Here's how the part is built. I have some questions about the finished solid (model axes, mm). A direction names the side the tool comes from. Round coordinates to 2 decimals unless told otherwise and drop trailing zeros. Order: outer loops, then holes, each group sorted by start corner. A loop starts at its lowest first (then second) coordinate and runs counter-clockwise, first axis right, second up.
```python
from build123d import *

# Parameters (mm, degrees)
SKETCH_1_W          = 350
SKETCH_1_H          = 50
SKETCH_1_R          = 2.75
EXTRUDE_1_DEPTH     = 5
SKETCH_2_W          = 350
SKETCH_2_H          = 6
EXTRUDE_2_DEPTH     = 364
SKETCH_3_R          = 2.75
CUT_EXTRUDE_1_DEPTH = 500
SKETCH_4_R          = 1.75
CUT_EXTRUDE_2_DEPTH = 10
FILLET_1_R          = 20
SKETCH_5_R          = 1.75
CUT_EXTRUDE_3_DEPTH = 10


with BuildPart() as part:
    # 草图1 → 凸台-拉伸1 (new body)
    with BuildSketch(Plane(origin=(0, 0, 0), x_dir=(1, 0, 0), z_dir=(0, 1, 0))):
        with Locations((0, 25)):
            Rectangle(SKETCH_1_W, SKETCH_1_H)
        with Locations(Location((130, 25, 0), (0, 0, 270))):
            Circle(SKETCH_1_R, mode=Mode.SUBTRACT)
        with Locations(Location((50, 25, 0), (0, 0, 270))):
            Circle(SKETCH_1_R, mode=Mode.SUBTRACT)
        with Locations(Location((-130, 25, 0), (0, 0, 90))):
            Circle(SKETCH_1_R, mode=Mode.SUBTRACT)
        with Locations(Location((-50, 25, 0), (0, 0, 90))):
            Circle(SKETCH_1_R, mode=Mode.SUBTRACT)
    extrude(amount=EXTRUDE_1_DEPTH)

    # 草图2 → 凸台-拉伸2 (add)
    with BuildSketch(Plane(origin=(0, 5, 0), x_dir=(1, 0, 0), z_dir=(0, 1, 0))):
        with Locations((0, 3)):
            Rectangle(SKETCH_2_W, SKETCH_2_H)
    extrude(amount=EXTRUDE_2_DEPTH)

    # 草图3 → 切除-拉伸1 (cut)
    with BuildSketch(Plane(origin=(0, 0, -6), x_dir=(-1, 0, 0), z_dir=(0, 0, -1))):
        with Locations((87.5, 274)):
            Circle(SKETCH_3_R)
        with Locations((87.5, 124)):
            Circle(SKETCH_3_R)
        with Locations((-87.5, 124)):
            Circle(SKETCH_3_R)
        with Locations((-87.5, 274)):
            Circle(SKETCH_3_R)
        with Locations((152.5, 339)):
            Circle(SKETCH_3_R)
        with Locations((152.5, 189)):
            Circle(SKETCH_3_R)
        with Locations((152.5, 39)):
            Circle(SKETCH_3_R)
        with Locations((-152.5, 39)):
            Circle(SKETCH_3_R)
        with Locations((-152.5, 189)):
            Circle(SKETCH_3_R)
        with Locations((-152.5, 339)):
            Circle(SKETCH_3_R)
        with Locations((0, 339)):
            Circle(SKETCH_3_R)
        with Locations((0, 189)):
            Circle(SKETCH_3_R)
        with Locations((0, 39)):
            Circle(SKETCH_3_R)
        with BuildLine():
            Line((83.964466094, 137.535533906), (41.035533906, 180.464466094))
            ThreePointArc((41.035533906, 180.464466094), (39.951670149, 185.913417162), (44.571067812, 189))
            Line((44.571067812, 189), (130.428932188, 189))
            ThreePointArc((130.428932188, 189), (135.048329851, 185.913417162), (133.964466094, 180.464466094))
            Line((133.964466094, 180.464466094), (91.035533906, 137.535533906))
            ThreePointArc((91.035533906, 137.535533906), (87.5, 136.071067812), (83.964466094, 137.535533906))
        make_face()
        with BuildLine():
            Line((44.571067812, 339), (130.428932188, 339))
            ThreePointArc((130.428932188, 339), (135.048329851, 335.913417162), (133.964466094, 330.464466094))
            Line((133.964466094, 330.464466094), (91.035533906, 287.535533906))
            ThreePointArc((91.035533906, 287.535533906), (87.5, 286.071067812), (83.964466094, 287.535533906))
            Line((83.964466094, 287.535533906), (41.035533906, 330.464466094))
            ThreePointArc((41.035533906, 330.464466094), (39.951670149, 335.913417162), (44.571067812, 339))
        make_face()
        with BuildLine():
            Line((73.964466094, 120.464466094), (31.035533906, 77.535533906))
            ThreePointArc((31.035533906, 77.535533906), (25.586582838, 76.451670149), (22.5, 81.071067812))
            Line((22.5, 81.071067812), (22.5, 166.928932188))
            ThreePointArc((22.5, 166.928932188), (25.586582838, 171.548329851), (31.035533906, 170.464466094))
            Line((31.035533906, 170.464466094), (73.964466094, 127.535533906))
            ThreePointArc((73.964466094, 127.535533906), (75.428932188, 124), (73.964466094, 120.464466094))
        make_face()
        with BuildLine():
            Line((101.035533906, 277.535533906), (143.964466094, 320.464466094))
            ThreePointArc((143.964466094, 320.464466094), (149.413417162, 321.548329851), (152.5, 316.928932188))
            Line((152.5, 316.928932188), (152.5, 231.071067812))
            ThreePointArc((152.5, 231.071067812), (149.413417162, 226.451670149), (143.964466094, 227.535533906))
            Line((143.964466094, 227.535533906), (101.035533906, 270.464466094))
            ThreePointArc((101.035533906, 270.464466094), (99.571067812, 274), (101.035533906, 277.535533906))
        make_face()
        with BuildLine():
            Line((91.035533906, 260.464466094), (133.964466094, 217.535533906))
            ThreePointArc((133.964466094, 217.535533906), (135.048329851, 212.086582838), (130.428932188, 209))
            Line((130.428932188, 209), (44.571067812, 209))
            ThreePointArc((44.571067812, 209), (39.951670149, 212.086582838), (41.035533906, 217.535533906))
            Line((41.035533906, 217.535533906), (83.964466094, 260.464466094))
            ThreePointArc((83.964466094, 260.464466094), (87.5, 261.928932188), (91.035533906, 260.464466094))
        make_face()
        with BuildLine():
            Line((73.964466094, 270.464466094), (31.035533906, 227.535533906))
            ThreePointArc((31.035533906, 227.535533906), (25.586582838, 226.451670149), (22.5, 231.071067812))
            Line((22.5, 231.071067812), (22.5, 316.928932188))
            ThreePointArc((22.5, 316.928932188), (25.586582838, 321.548329851), (31.035533906, 320.464466094))
            Line((31.035533906, 320.464466094), (73.964466094, 277.535533906))
            ThreePointArc((73.964466094, 277.535533906), (75.428932188, 274), (73.964466094, 270.464466094))
        make_face()
        with BuildLine():
            Line((101.035533906, 127.535533906), (143.964466094, 170.464466094))
            ThreePointArc((143.964466094, 170.464466094), (149.413417162, 171.548329851), (152.5, 166.928932188))
            Line((152.5, 166.928932188), (152.5, 81.071067812))
            ThreePointArc((152.5, 81.071067812), (149.413417162, 76.451670149), (143.964466094, 77.535533906))
            Line((143.964466094, 77.535533906), (101.035533906, 120.464466094))
            ThreePointArc((101.035533906, 120.464466094), (99.571067812, 124), (101.035533906, 127.535533906))
        make_face()
        with BuildLine():
            Line((91.035533906, 110.464466094), (133.964466094, 67.535533906))
            ThreePointArc((133.964466094, 67.535533906), (135.048329851, 62.086582838), (130.428932188, 59))
            Line((130.428932188, 59), (44.571067812, 59))
            ThreePointArc((44.571067812, 59), (39.951670149, 62.086582838), (41.035533906, 67.535533906))
            Line((41.035533906, 67.535533906), (83.964466094, 110.464466094))
            ThreePointArc((83.964466094, 110.464466094), (87.5, 111.928932188), (91.035533906, 110.464466094))
        make_face()
        with BuildLine():
            Line((-91.035533906, 137.535533906), (-133.964466094, 180.464466094))
            ThreePointArc((-133.964466094, 180.464466094), (-135.048329851, 185.913417162), (-130.428932188, 189))
            Line((-130.428932188, 189), (-44.571067812, 189))
            ThreePointArc((-44.571067812, 189), (-39.951670149, 185.913417162), (-41.035533906, 180.464466094))
            Line((-41.035533906, 180.464466094), (-83.964466094, 137.535533906))
            ThreePointArc((-83.964466094, 137.535533906), (-87.5, 136.071067812), (-91.035533906, 137.535533906))
        make_face()
        with BuildLine():
            Line((-101.035533906, 120.464466094), (-143.964466094, 77.535533906))
            ThreePointArc((-143.964466094, 77.535533906), (-149.413417162, 76.451670149), (-152.5, 81.071067812))
            Line((-152.5, 81.071067812), (-152.5, 166.928932188))
            ThreePointArc((-152.5, 166.928932188), (-149.413417162, 171.548329851), (-143.964466094, 170.464466094))
            Line((-143.964466094, 170.464466094), (-101.035533906, 127.535533906))
            ThreePointArc((-101.035533906, 127.535533906), (-99.571067812, 124), (-101.035533906, 120.464466094))
        make_face()
        with BuildLine():
            Line((-73.964466094, 127.535533906), (-31.035533906, 170.464466094))
            ThreePointArc((-31.035533906, 170.464466094), (-25.586582838, 171.548329851), (-22.5, 166.928932188))
            Line((-22.5, 166.928932188), (-22.5, 81.071067812))
            ThreePointArc((-22.5, 81.071067812), (-25.586582838, 76.451670149), (-31.035533906, 77.535533906))
            Line((-31.035533906, 77.535533906), (-73.964466094, 120.464466094))
            ThreePointArc((-73.964466094, 120.464466094), (-75.428932188, 124), (-73.964466094, 127.535533906))
        make_face()
        with BuildLine():
            Line((-83.964466094, 110.464466094), (-41.035533906, 67.535533906))
            ThreePointArc((-41.035533906, 67.535533906), (-39.951670149, 62.086582838), (-44.571067812, 59))
            Line((-44.571067812, 59), (-130.428932188, 59))
            ThreePointArc((-130.428932188, 59), (-135.048329851, 62.086582838), (-133.964466094, 67.535533906))
            Line((-133.964466094, 67.535533906), (-91.035533906, 110.464466094))
            ThreePointArc((-91.035533906, 110.464466094), (-87.5, 111.928932188), (-83.964466094, 110.464466094))
        make_face()
        with BuildLine():
            Line((-91.035533906, 287.535533906), (-133.964466094, 330.464466094))
            ThreePointArc((-133.964466094, 330.464466094), (-135.048329851, 335.913417162), (-130.428932188, 339))
            Line((-130.428932188, 339), (-44.571067812, 339))
            ThreePointArc((-44.571067812, 339), (-39.951670149, 335.913417162), (-41.035533906, 330.464466094))
            Line((-41.035533906, 330.464466094), (-83.964466094, 287.535533906))
            ThreePointArc((-83.964466094, 287.535533906), (-87.5, 286.071067812), (-91.035533906, 287.535533906))
        make_face()
        with BuildLine():
            Line((-101.035533906, 270.464466094), (-143.964466094, 227.535533906))
            ThreePointArc((-143.964466094, 227.535533906), (-149.413417162, 226.451670149), (-152.5, 231.071067812))
            Line((-152.5, 231.071067812), (-152.5, 316.928932188))
            ThreePointArc((-152.5, 316.928932188), (-149.413417162, 321.548329851), (-143.964466094, 320.464466094))
            Line((-143.964466094, 320.464466094), (-101.035533906, 277.535533906))
            ThreePointArc((-101.035533906, 277.535533906), (-99.571067812, 274), (-101.035533906, 270.464466094))
        make_face()
        with BuildLine():
            Line((-73.964466094, 277.535533906), (-31.035533906, 320.464466094))
            ThreePointArc((-31.035533906, 320.464466094), (-25.586582838, 321.548329851), (-22.5, 316.928932188))
            Line((-22.5, 316.928932188), (-22.5, 231.071067812))
            ThreePointArc((-22.5, 231.071067812), (-25.586582838, 226.451670149), (-31.035533906, 227.535533906))
            Line((-31.035533906, 227.535533906), (-73.964466094, 270.464466094))
            ThreePointArc((-73.964466094, 270.464466094), (-75.428932188, 274), (-73.964466094, 277.535533906))
        make_face()
        with BuildLine():
            Line((-83.964466094, 260.464466094), (-41.035533906, 217.535533906))
            ThreePointArc((-41.035533906, 217.535533906), (-39.951670149, 212.086582838), (-44.571067812, 209))
            Line((-44.571067812, 209), (-130.428932188, 209))
            ThreePointArc((-130.428932188, 209), (-135.048329851, 212.086582838), (-133.964466094, 217.535533906))
            Line((-133.964466094, 217.535533906), (-91.035533906, 260.464466094))
            ThreePointArc((-91.035533906, 260.464466094), (-87.5, 261.928932188), (-83.964466094, 260.464466094))
        make_face()
    extrude(amount=-CUT_EXTRUDE_1_DEPTH, mode=Mode.SUBTRACT)

    # 草图4 → 切除-拉伸2 (cut)
    with BuildSketch(Plane.XY):
        with Locations((60, 366)):
            Circle(SKETCH_4_R)
        with Locations((85, 366)):
            Circle(SKETCH_4_R)
        with Locations((12.5, 366)):
            Circle(SKETCH_4_R)
        with Locations((-12.5, 366)):
            Circle(SKETCH_4_R)
        with Locations((-85, 366)):
            Circle(SKETCH_4_R)
        with Locations((-60, 366)):
            Circle(SKETCH_4_R)
    extrude(amount=-CUT_EXTRUDE_2_DEPTH, mode=Mode.SUBTRACT)

    # 圆角1
    fillet_1_edges = [part.edges().sort_by_distance(p)[0] for p in [
        (-175, 369, -3),
        (175, 369, -3),
    ]]
    fillet(fillet_1_edges, radius=FILLET_1_R)

    # 草图5 → 切除-拉伸3 (cut)
    with BuildSketch(Plane(origin=(0, 0, -6), x_dir=(-1, 0, 0), z_dir=(0, 0, -1))):
        with Locations((172, 330)):
            Circle(SKETCH_5_R)
        with Locations((172, 230)):
            Circle(SKETCH_5_R)
        with Locations((-172, 230)):
            Circle(SKETCH_5_R)
        with Locations((-172, 330)):
            Circle(SKETCH_5_R)
    extrude(amount=-CUT_EXTRUDE_3_DEPTH, mode=Mode.SUBTRACT)


solid = part.part
```
1. I'm going to push flat-ended pins straight in: P1, Ø3, axis at x = 118, y = 212, coming from the -Z side; P2, Ø3, axis at x = 28, z = -32.5, coming from the +Y side; P3, Ø3, axis at x = 71, y = 298.5, coming from the -Z side. Where does each tip first touch, or does it pass through?
Evaluation:
P1: passes through
P2: stops at y = 5
P3: stops at z = -6
2. I need wall thicknesses on probe 1 along X at (y, z) = (2, -25); probe 2 along Y at (x, z) = (-12.5, -3.25); probe 3 along Z at (x, y) = (-144, 172.5). Which ranges of each line are inside material? Lowest first, please.
Evaluation:
probe 1: x = -175 to -132.75, -127.25 to -52.75, -47.25 to 47.25, 52.75 to 127.25, 132.75 to 175
probe 2: y = 0 to 364.25, 367.75 to 369
probe 3: z = -6 to 0
3. If we section it at B-B, the plane z = -36: Write out the boundary of the cut face in (x, y).
Evaluation:
outline: (-175, 0) - (175, 0) - (175, 5) - (-175, 5) - close
4. If we section it at A-A, the plane y = 152.5: Write out the boundary of the cut face in (x, z).
Evaluation:
outline: (-175, -6) - (-152.5, -6) - (-152.5, 0) - (-175, 0) - close; (-126, -6) - (-106, -6) - (-106, 0) - (-126, 0) - close; (-69, -6) - (-49, -6) - (-49, 0) - (-69, 0) - close; (-22.5, -6) - (22.5, -6) - (22.5, 0) - (-22.5, 0) - close; (49, -6) - (69, -6) - (69, 0) - (49, 0) - close; (106, -6) - (126, -6) - (126, 0) - (106, 0) - close; (152.5, -6) - (175, -6) - (175, 0) - (152.5, 0) - close
5. On a 3-axis mill with a long thin cutter (end or side, diameter ignored), from which of +Z, -Z, +X, -X, +Y, -Y can I reach the whole of each face in a straight line? I mean faces 1 (the flat face through (62.2, 309.3, -3)), 2 (the flat face through (-2, 184, -6)). Say none if no direction works.
Evaluation:
face 1: +Z, -Z
face 2: -Z, +X, -X, +Y
6. If we mould it in two halves opening along X, with no side actions, what happens to faces 3 (the cylindrical face through (-169.297, 362.986, -3.042)), 4 (the flat face through (175, 174, -3)), 5 (the flat face through (-122.2, 298.7, -3))? For each: released by +X, released by -X, zero draft, split by the parting line, or undercut.
Evaluation:
face 3: released by -X
face 4: released by +X
face 5: undercut
